```python
from build123d import *

# Parameters (mm, degrees)
SKETCH_1_W                  = 7
SKETCH_1_H                  = 44
EXTRUDE_485_DEPTH           = 12.5
FILLET_3_R                  = 1.5
CUT_EXTRUDE_1218_REACH      = 28.254
SKETCH_6_R                  = 4
CUT_EXTRUDE_1261_REACH      = 28.254
SKETCH_7_W                  = 6.25
SKETCH_7_H                  = 18
SKETCH_11_R                 = 1.15
CUT_EXTRUDE_1309_DEPTH      = 8
CUT_EXTRUDE_1453_DEPTH      = 2.2
CUT_EXTRUDE_1453_DEPTH_BACK = 2.2
SKETCH_12_R                 = 5.25
SKETCH_13_R                 = 0.75
CUT_EXTRUDE_1751_DEPTH      = 5.5
CHAMFER_1_SIZE              = 0.75


with BuildPart() as part:
    # Эскиз1 → Extrude 485 (new body)
    with BuildSketch(Plane.XY):
        Rectangle(SKETCH_1_W, SKETCH_1_H)
    extrude(amount=EXTRUDE_485_DEPTH)

    # Скругление3
    fillet_3_edges = [part.edges().sort_by_distance(p)[0] for p in [
        (-3.5, 0, 12.5),
        (-3.5, 0, 0),
    ]]
    fillet(fillet_3_edges, radius=FILLET_3_R)

    # Эскиз6 → Cut-Extrude 1218 (cut, up to next)
    with BuildSketch(Plane.ZY.offset(3.5), mode=Mode.PRIVATE) as cut_extrude_1218_sk1:
        with Locations((6.25, -3.5)):
            Circle(SKETCH_6_R)
    cut_extrude_1218_tool1 = extrude(cut_extrude_1218_sk1.sketch, amount=-CUT_EXTRUDE_1218_REACH, mode=Mode.PRIVATE) & part.part
    add(cut_extrude_1218_tool1.solids().sort_by_distance((-3.5, -3.5, 6.25))[0], mode=Mode.SUBTRACT)

    # Эскиз7 → Cut-Extrude 1261 (cut, up to next)
    with BuildSketch(Plane.ZY.offset(3.5), mode=Mode.PRIVATE) as cut_extrude_1261_sk1:
        with Locations((9.375, -3.5)):
            Rectangle(SKETCH_7_W, SKETCH_7_H)
    cut_extrude_1261_tool1 = extrude(cut_extrude_1261_sk1.sketch, amount=-CUT_EXTRUDE_1261_REACH, mode=Mode.PRIVATE) & part.part
    add(cut_extrude_1261_tool1.solids().sort_by_distance((-3.5, -3.5, 9.375))[0], mode=Mode.SUBTRACT)

    # Эскиз11 → Cut-Extrude 1309 (cut)
    with BuildSketch(Plane.XZ.offset(22)):
        with Locations(Location((0, 6.25, 0), (0, 0, 270))):
            Circle(SKETCH_11_R)
    cut_extrude_1309 = extrude(amount=-CUT_EXTRUDE_1309_DEPTH, mode=Mode.SUBTRACT)

    # Mirror 1353: Cut-Extrude 1309 across plane
    add(cut_extrude_1309.mirror(Plane.ZX), mode=Mode.SUBTRACT)

    # Эскиз12 → Cut-Extrude 1453 (cut, two sides: drawn at the far end of the back side and taken through both)
    with BuildSketch(Plane(origin=(0, 0, 0), x_dir=(0, 0, -1), z_dir=(1, 0, 0)).offset(-CUT_EXTRUDE_1453_DEPTH_BACK)):
        with Locations((-6.25, -3.5)):
            Circle(SKETCH_12_R)
    extrude(amount=CUT_EXTRUDE_1453_DEPTH + CUT_EXTRUDE_1453_DEPTH_BACK, mode=Mode.SUBTRACT)

    # Эскиз13 → Cut-Extrude 1751 (cut)
    with BuildSketch(Plane.XY.offset(6.25)):
        with Locations((0, 3.5)):
            Circle(SKETCH_13_R)
        with Locations((0, -10.5)):
            Circle(SKETCH_13_R)
    extrude(amount=-CUT_EXTRUDE_1751_DEPTH, mode=Mode.SUBTRACT)

    # Фаска1
    chamfer_1_edges = [part.edges().sort_by_distance(p)[0] for p in [
        (-3.5, -3.5, 2.25),
        (3.5, -3.5, 2.25),
    ]]
    chamfer(chamfer_1_edges, length=CHAMFER_1_SIZE - 0.0001)  # a hair under: the kernel refuses the full size


solid = part.part
```
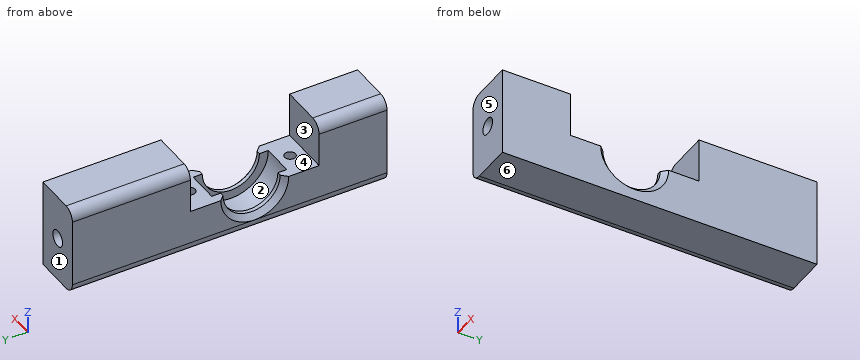
Source: CAD feature listing. Evaluate the final solid. Frame: model axes, mm. Face numbers are marked on the shaded views. A direction names the side the tool comes from. Round coordinates to 2 decimals unless told otherwise and drop trailing zeros. Order: outer loops, then holes, each group sorted by start corner. A loop starts at its lowest first (then second) coordinate and runs counter-clockwise, first axis right, second up. Notation, with made-up numbers: (13, 71) -> (36, 71) arc R20 ccw to (36, 101) -> close; hole circle Ø7 at (-17.75, 23.5). An arc over 180 degrees is marked (long way). One line per item, written item: value. Start each with the question number.
Q1. Section query A-A (x = 0). Return the cut outline in (y, z).
Q2. Pin query (flat end, axial travel): pin 1 (1.6 mm diameter, centred on y = -3, z = 4, fed in from +X); pin 2 (1.7 mm diameter, centred on x = 0, y = -10.5, fed in from +Z); pin 3 (2 mm diameter, centred on x = 0, z = 6.25, fed in from +Y); pin 4 (0.7 mm diameter, centred on x = -0.5, z = 6.5, fed in from -Y). Return the tip coordinate at first contact, or that it passes through.
Q3. Material intervals for probe 1 along Y at (x, z) = (-0.5, 7.5); probe 2 along Y at (x, z) = (0, 3.5); probe 3 along Y at (x, z) = (0, 6), sorted ascending.
Q4. Draft query along Y for the marked faces 4, 5 and 6. Return one class per face: pulls with the +Y half, pulls with the -Y half, needs draft (parallel to the pull), parting line crosses it, or undercut.
Q5. Access query for the marked faces 1, 2 and 3. Directions: +Z, -Z, +X, -X, +Y, -Y. A direction counts if a zero-diameter tool reaches every point of the face in a straight line with its end or side. Return the directions, or none.
Q6. Section query C-C (y = 3.5). Return the cut outline in (x, z).
Q7. Section query B-B (y = -18.5). Return the cut outline in (x, z), plus the area to 3 significant figures.
Findings below:
1. outline: (-22, 0) -> (22, 0) -> (22, 5.1) -> (14, 5.1) -> (14, 7.4) -> (22, 7.4) -> (22, 12.5) -> (5.5, 12.5) -> (5.5, 6.25) -> (4.25, 6.25) -> (4.25, 0.75) -> (2.75, 0.75) -> (2.75, 6.25) -> (1.75, 6.25) arc R5.25 cw to (-8.75, 6.25) -> (-9.75, 6.25) -> (-9.75, 0.75) -> (-11.25, 0.75) -> (-11.25, 6.25) -> (-12.5, 6.25) -> (-12.5, 12.5) -> (-22, 12.5) -> (-22, 7.4) -> (-14, 7.4) -> (-14, 5.1) -> (-22, 5.1) -> close
2. pin 1: through
2. pin 2: z = 6.25
2. pin 3: y = 14
2. pin 4: y = -14
3. probe 1: -22 to -12.5, 5.5 to 22
3. probe 2: -22 to -11.25, -9.75 to -7.97, 0.97 to 2.75, 4.25 to 22
3. probe 3: -14 to -11.25, -9.75 to -8.74, 1.74 to 2.75, 4.25 to 14
4. face 4: undercut
4. face 5: pulls with the -Y half
4. face 6: needs draft
5. face 1: +Z, -Z, +X, -X, +Y
5. face 2: +Z
5. face 3: +Z, +X, -X
6. outline: (-3.5, 1.5) arc R1.5 ccw to (-2, 0) -> (3.5, 0) -> (3.5, 6.25) -> (0.75, 6.25) -> (0.75, 0.75) -> (-0.75, 0.75) -> (-0.75, 6.25) -> (-3.5, 6.25) -> close
7. outline: (-3.5, 1.5) arc R1.5 ccw to (-2, 0) -> (3.5, 0) -> (3.5, 12.5) -> (-2, 12.5) arc R1.5 ccw to (-3.5, 11) -> close; hole circle Ø2.3 at (0, 6.25)
7. area: 82.4 mm²
